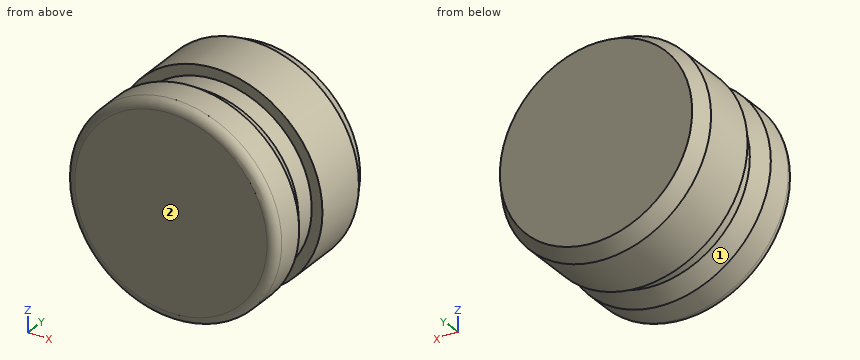
```python
from build123d import *

# Parameters (mm, degrees)
FILLET1_R      = 0.79375
CHAMFER1_SIZE  = 0.79375
CHAMFER1_SIZE2 = 1.374815329


with BuildPart() as part:
    # Sketch1 → Revolve1 (revolve)
    with BuildSketch(Plane.XY):
        Polygon((0, 0), (-9.4234, 0), (-9.4234, 3.175), (-8.4582, 4.572), (-8.4582, 6.35), (-9.4234, 6.35), (-9.4234, 12.7), (0, 12.7), align=None)
    revolve(axis=Axis((0, 0, 0), (0, 1, 0)))

    # Fillet1
    fillet1_edges = [part.edges().sort_by_distance(p)[0] for p in [
        (9.4234, 0, 0),
    ]]
    fillet(fillet1_edges, radius=FILLET1_R)

    # Chamfer1
    chamfer1_edges = [part.edges().sort_by_distance(p)[0] for p in [
        (9.4234, 12.7, 0),
    ]]
    chamfer1_side = [part.faces().sort_by_distance(p)[0] for p in [
        (0, 12.7, 0),
    ]]
    chamfer(chamfer1_edges, length=CHAMFER1_SIZE, length2=CHAMFER1_SIZE2, reference=chamfer1_side[0])


solid = part.part
```
Source: CAD feature listing. Evaluate the final solid. Frame: model axes, mm. Face numbers are marked on the shaded views. Give positions to 0.01 mm unless a question says otherwise; leave off trailing zeros. Write each loop counter-clockwise with the first axis right and the second up, starting at its lowest first coordinate (ties: lowest second). Pieces come first, ordered by that corner, then holes. Notation, with made-up numbers: (76.25, 13.25) - (83.25, 13.25) arc R22 cw to (83.25, 33.25) - close; hole circle Ø9 at (85, 86.25). An arc over 180 degrees is marked (long way). One line per item, written item: value. Start each with the question number.
Q1. Material intervals for probe 1 along Y at (x, z) = (-7, 5.75); probe 2 along X at (y, z) = (3, 4.5); probe 3 along X at (y, z) = (10.5, -0.25), sorted ascending. Write a range as from..to.
Q2. Section query C-C, the plane y = 7. Return the cut outline in (x, z), then the cut area to 3 significant figures.
Q3. Draft query along Z for the marked faces 1 and 2. Return one class per face: +Z half, -Z half, draft (parallel to the pull), parting line (faces both ways), or undercut.
Q4. First-contact query: pin 1 Ø1.5 at (x, y) = (7.5, 6.5) entering from +Z; pin 2 Ø4 at (x, y) = (2.5, 4.5) entering from +Z; pin 3 Ø6 at (y, z) = (9.5, 4.5) entering from +X. Flat tips, straight axial feed; report the tip coordinate or a pass-through.
Answer:
1. probe 1: y = 0.13..3.7, 6.35..11.96
1. probe 2: x = -8.28..8.28
1. probe 3: x = -9.42..9.42
2. outline: circle Ø18.85 at (0, 0)
2. area: 279 mm2
3. face 1: parting line
3. face 2: draft
4. pin 1: stops at z = 6.58
4. pin 2: stops at z = 9.37
4. pin 3: stops at x = 9.3
